Work out the finished part from the listing and answer in its coordinate system (mm). Round coordinates to 2 decimals unless told otherwise and drop trailing zeros. Order: outer loops, then holes, each group sorted by start corner. A loop starts at its lowest first (then second) coordinate and runs counter-clockwise, first axis right, second up. Notation, with made-up numbers: (-38.75, -14) - (-8.75, -14) arc R29 ccw to (-8.75, 17) - close; hole circle Ø4 at (15, -31.75). An arc over 180 degrees is marked (long way). Use one line per item in the form item = value. Start each with the question number.
Q1. The part is cut by section A-A on x = 0. Determine the outline of the cut face in (y, z).
Q2. The part is cut by section B-B on y = 0. Determine the outline of the cut face in (x, z) (3 decimals).
Q3. The part is cut by section C-C on z = 17. Determine the outline of the cut face in (x, y) (3 decimals).
Q4. Find the intervals of material crossed by line 1 (Y direction, x = -1.5, z = 62); line 2 (Z direction, x = -1, y = 0.75); line 3 (Z direction, x = -1.5, y = 1), in increasing order. Write a range as [from, to].
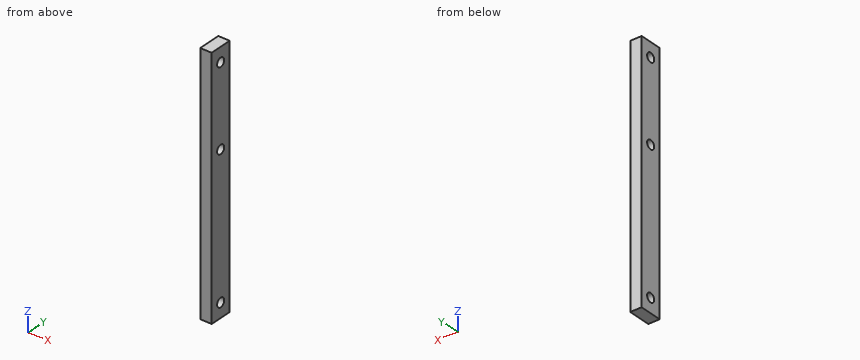
from build123d import *

# Parameters (mm, degrees)
BOSS_EXTRUDE1_DEPTH      = 70
BOSS_EXTRUDE1_DEPTH_BACK = 70
SKETCH2_W                = 6.35
SKETCH2_H                = 12.7
SKETCH4_R                = 2.5
CUT_EXTRUDE1_DEPTH       = 71.573684897


with BuildPart() as part:
    # Sketch2 → Boss-Extrude1 (new, two sides: drawn at the far end of the back side and taken through both)
    with BuildSketch(Plane.XY.offset(-BOSS_EXTRUDE1_DEPTH_BACK)):
        Rectangle(SKETCH2_W, SKETCH2_H)
    extrude(amount=BOSS_EXTRUDE1_DEPTH + BOSS_EXTRUDE1_DEPTH_BACK)

    # Sketch4 → Cut-Extrude1 (cut, through all)
    with BuildSketch(Plane(origin=(3.175, 0, 0), x_dir=(0, 0, -1), z_dir=(1, 0, 0))):
        with Locations((-62, 0)):
            Circle(SKETCH4_R)
        with Locations(Location((62, 0, 0), (0, 0, 180))):
            Circle(SKETCH4_R)
        with Locations((-17, 0)):
            Circle(SKETCH4_R)
    extrude(amount=-CUT_EXTRUDE1_DEPTH, mode=Mode.SUBTRACT)


solid = part.part
Found:
q1.outline = (-6.35, -70) - (6.35, -70) - (6.35, 70) - (-6.35, 70) - close; hole circle Ø5 at (0, -62); hole circle Ø5 at (0, 17); hole circle Ø5 at (0, 62)
q2.outline = (-3.175, -70) - (3.175, -70) - (3.175, -64.5) - (-3.175, -64.5) - close; (-3.175, -59.5) - (3.175, -59.5) - (3.175, 14.5) - (-3.175, 14.5) - close; (-3.175, 19.5) - (3.175, 19.5) - (3.175, 59.5) - (-3.175, 59.5) - close; (-3.175, 64.5) - (3.175, 64.5) - (3.175, 70) - (-3.175, 70) - close
q3.outline = (-3.175, -6.35) - (3.175, -6.35) - (3.175, -2.5) - (-3.175, -2.5) - close; (-3.175, 2.5) - (3.175, 2.5) - (3.175, 6.35) - (-3.175, 6.35) - close
q4.line_1 = [-6.35, -2.5], [2.5, 6.35]
q4.line_2 = [-70, -64.38], [-59.62, 14.62], [19.38, 59.62], [64.38, 70]
q4.line_3 = [-70, -64.29], [-59.71, 14.71], [19.29, 59.71], [64.29, 70]
